Autodesk Inventor part; units mm, degrees
ref_plane "YZ Plane" through (0, 0, 0) normal (1, 0, 0) x (0, 1, 0)
ref_plane "XZ Plane" through (0, 0, 0) normal (0, 1, 0) x (-1, 0, 0)
ref_plane "XY Plane" through (0, 0, 0) normal (0, 0, 1) x (1, 0, 0)
sketch "Эскиз1" plane through (0, 0, 0) normal (0, 0, 1) x (1, 0, 0)
  line L0 (-177.5, 105) -> (177.5, 105)
  line L1 (177.5, 105) -> (177.5, -105)
  line L2 (177.5, -105) -> (-177.5, -105)
  line L3 (-177.5, -105) -> (-177.5, 105)
  line L4 (-177.5, 105) -> (177.5, -105) construction
  line L5 (177.5, 105) -> (-177.5, -105) construction
  point P0 (0, 0)
  dimension "d0" = 355
  dimension "d1" = 210
extrude "Выдавливание1" add sketch "Эскиз1" along normal blind 4
sketch "Эскиз2" plane through (0, 0, 4) normal (0, 0, 1) x (1, 0, 0)
  line L0 (-177.5, -105) -> (177.5, -105)
  line L1 (177.5, -105) -> (177.5, 105)
  line L2 (-177.5, -105) -> (177.5, -105)
  line L3 (177.5, -105) -> (177.5, -45)
  line L4 (177.5, -45) -> (-177.5, -45)
  line L5 (-177.5, -45) -> (-177.5, -105)
  point P0 (0, 0)
  dimension "d4" = 60
extrude "Выдавливание2" add sketch "Эскиз2" along normal blind 4
sketch "Эскиз3" plane through (0, 0, 4) normal (0, 0, 1) x (1, 0, 0)
  circle A0 centre (-162.5, 90) radius 15
  circle A1 centre (162.5, -30) radius 15
  line L0 (177.5, 105) -> (-177.5, 105) construction
  line L1 (-177.5, 105) -> (-177.5, -45) construction
  line L2 (177.5, -45) -> (-177.5, -45) construction
  line L3 (177.5, -45) -> (177.5, 105) construction
  circle A2 centre (-162.5, 90) radius 12.75
  circle A3 centre (162.5, -30) radius 12.75
  point P0 (0, 0)
  dimension "d14" = 30
  dimension "d15" = 30
  dimension "d16" = 25.5
  dimension "d17" = 25.5
extrude "Выдавливание3" add sketch "Эскиз3" along normal blind 2 contours A2 | A3
properties part number "монитор"
Geometry check sheet. Reference: the model listing, model coordinates, mm. A direction names the side the tool comes from. Round coordinates to 2 decimals unless told otherwise and drop trailing zeros. Loops run counter-clockwise (first coordinate to the right, second up) from the corner with the lowest first, then second, coordinate; pieces in that order, holes last. Notation, with made-up numbers: M -23,46 L 35,46 A19 ccw 35,62 Z; hole C -17.5,-35.75 d6. An arc over 180 degrees is marked long. Return JSON: item names as keys, results as strings. Group by question number.
(1) Set-up check for faces 1 (the face through (-2, 1, 0)), 2 (the face through (-172.618, 97.758, 4.986)), 3 (the face through (162, -30, 6)): record each of +Z, -Z, +X, -X, +Y, -Y from which the full face is reachable in a straight line by a thin tool's end or side.
(2) Section check C-C, the plane y = 41. Enter the section's corners in (x, z), and give its area (3 significant figures).
(3) Go/stop test with flat-tipped pins: pin 1 (20.5 mm diameter, centred on x = 162.5, y = -31, fed in from +Z); pin 2 (12 mm diameter, centred on x = 42.5, y = 65.5, fed in from +Z); pin 3 (2 mm diameter, centred on y = 71.5, z = 6.5, fed in from +X); pin 4 (1.2 mm diameter, centred on x = 31.5, z = 5.5, fed in from +Y). Record where each tip stops, or that it passes through.
(4) Section check A-A, the plane y = 90. Enter the section's corners in (x, z), and give its area (3 significant figures).
(5) Mould release check, pull along Y, two halves, no side actions. Record for faces 4 (the face through (-177.5, -25, 3)), 5 (the face through (2, -105, 4)), 6 (the face through (152.382, -22.242, 4.986)): pulls with the +Y half, pulls with the -Y half, needs draft (parallel to the pull), parting line crosses it, or undercut.
(6) Scan lines: line 1 along Z through (x, y) = (-40, 27); line 2 along Y through (x, z) = (-46, 6.25); line 3 along X through (y, z) = (95, 4.5). Record each from-to range of solid material in increasing order. Write a range as [from, to].
(7) Section check B-B, the plane x = -162.5. Enter the section's corners in (y, z), and give its area (3 significant figures).
Data:
{
 "1": {"face 1": "-Z, +X, -X, +Y, -Y", "face 2": "+Z", "face 3": "+Z, +X, -X, +Y"},
 "2": {"outline": "M -177.5,0 L 177.5,0 L 177.5,4 L -177.5,4 Z", "area": "1,420 mm²"},
 "3": {"pin 1": "z = 6", "pin 2": "z = 4", "pin 3": "through", "pin 4": "y = -45"},
 "4": {"outline": "M -177.5,0 L 177.5,0 L 177.5,4 L -149.75,4 L -149.75,6 L -175.25,6 L -175.25,4 L -177.5,4 Z", "area": "1,470 mm²"},
 "5": {"face 4": "needs draft", "face 5": "pulls with the -Y half", "face 6": "undercut"},
 "6": {"line 1": "[0, 4]", "line 2": "[-105, -45]", "line 3": "[-174.23, -150.77]"},
 "7": {"outline": "M -105,0 L 105,0 L 105,4 L 102.75,4 L 102.75,6 L 77.25,6 L 77.25,4 L -45,4 L -45,8 L -105,8 Z", "area": "1,130 mm²"}
}
